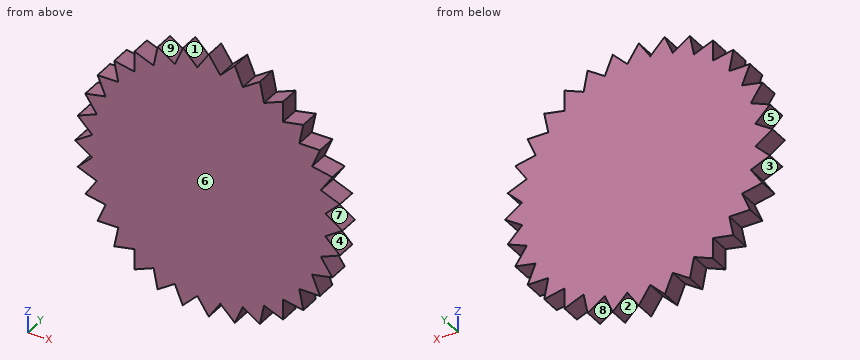
```python
from build123d import *

# Parameters (mm, degrees)
F1_DEPTH = 3.175


with BuildPart() as f1:
    # F0 (on Front) → F1 (new body, symmetric)
    with BuildSketch(Plane.XZ):
        Polygon((-23.3813293569, 34.9926322543), (-23.3813293569, 28.4902322543), (-17.3738950847, 32.5042715037), align=None)
        Polygon((-17.3738950847, 32.5042715037), (-23.3813293569, 28.4902322543), (-28.4902322543, 23.3813293569), (-32.5042715037, 17.3738950847), (-35.2691898278, 10.6987917678), (-36.678732966, 3.6125398832), (-36.678732966, -3.6125398832), (-35.2691898278, -10.6987917678), (-32.5042715037, -17.3738950847), (-28.4902322543, -23.3813293569), (-23.3813293569, -28.4902322543), (-17.3738950847, -32.5042715037), (-10.6987917678, -35.2691898278), (-3.6125398832, -36.678732966), (3.6125398832, -36.678732966), (10.6987917678, -35.2691898278), (17.3738950847, -32.5042715037), (23.3813293569, -28.4902322543), (28.4902322543, -23.3813293569), (32.5042715037, -17.3738950847), (35.2691898278, -10.6987917678), (36.678732966, -3.6125398832), (36.678732966, 3.6125398832), (35.2691898278, 10.6987917678), (32.5042715037, 17.3738950847), (28.4902322543, 23.3813293569), (23.3813293569, 28.4902322543), (17.3738950847, 32.5042715037), (10.6987917678, 35.2691898278), (3.6125398832, 36.678732966), (-3.6125398832, 36.678732966), (-10.6987917678, 35.2691898278), align=None)
        Polygon((-28.4902322543, 23.3813293569), (-23.3813293569, 28.4902322543), (-29.7587875642, 29.7587875642), align=None)
        Polygon((-16.1053397748, 38.881729711), (-17.3738950847, 32.5042715037), (-10.6987917678, 35.2691898278), align=None)
        Polygon((-32.5042715037, 17.3738950847), (-28.4902322543, 23.3813293569), (-34.9926322543, 23.3813293569), align=None)
        Polygon((-8.1233671151, 41.3620697513), (-10.6987917678, 35.2691898278), (-3.6125398832, 36.678732966), align=None)
        Polygon((-35.2691898278, 10.6987917678), (-32.5042715037, 17.3738950847), (-38.881729711, 16.1053397748), align=None)
        Polygon((0, 42.0852809731), (-3.6125398832, 36.678732966), (3.6125398832, 36.678732966), align=None)
        Polygon((-36.678732966, 3.6125398832), (-35.2691898278, 10.6987917678), (-41.2766241, 8.2104310172), align=None)
        Polygon((8.2104310172, 41.2766241), (3.6125398832, 36.678732966), (10.6987917678, 35.2691898278), align=None)
        Polygon((-36.678732966, -3.6125398832), (-36.678732966, 3.6125398832), (-42.0852809731, 0), align=None)
        Polygon((16.1053397748, 38.881729711), (10.6987917678, 35.2691898278), (17.3738950847, 32.5042715037), align=None)
        Polygon((-35.2691898278, -10.6987917678), (-36.678732966, -3.6125398832), (-41.2766241, -8.2104310172), align=None)
        Polygon((23.3813293569, 34.9926322543), (17.3738950847, 32.5042715037), (23.3813293569, 28.4902322543), align=None)
        Polygon((-32.5042715037, -17.3738950847), (-35.2691898278, -10.6987917678), (-38.881729711, -16.1053397748), align=None)
        Polygon((29.7587875642, 29.7587875642), (23.3813293569, 28.4902322543), (28.4902322543, 23.3813293569), align=None)
        Polygon((-28.4902322543, -23.3813293569), (-32.5042715037, -17.3738950847), (-34.9926322543, -23.3813293569), align=None)
        Polygon((34.9926322543, 23.3813293569), (28.4902322543, 23.3813293569), (32.5042715037, 17.3738950847), align=None)
        Polygon((-23.3813293569, -28.4902322543), (-28.4902322543, -23.3813293569), (-29.7587875642, -29.7587875642), align=None)
        Polygon((38.881729711, 16.1053397748), (32.5042715037, 17.3738950847), (35.2691898278, 10.6987917678), align=None)
        Polygon((-17.3738950847, -32.5042715037), (-23.3813293569, -28.4902322543), (-23.3813293569, -34.9926322543), align=None)
        Polygon((41.2766241, 8.2104310172), (35.2691898278, 10.6987917678), (36.678732966, 3.6125398832), align=None)
        Polygon((-10.6987917678, -35.2691898278), (-17.3738950847, -32.5042715037), (-16.1053397748, -38.881729711), align=None)
        Polygon((42.0852809731, 0), (36.678732966, 3.6125398832), (36.678732966, -3.6125398832), align=None)
        Polygon((-3.6125398832, -36.678732966), (-10.6987917678, -35.2691898278), (-8.2104310172, -41.2766241), align=None)
        Polygon((41.2766241, -8.2104310172), (36.678732966, -3.6125398832), (35.2691898278, -10.6987917678), align=None)
        Polygon((3.6125398832, -36.678732966), (-3.6125398832, -36.678732966), (0, -42.0852809731), align=None)
        Polygon((38.881729711, -16.1053397748), (35.2691898278, -10.6987917678), (32.5042715037, -17.3738950847), align=None)
        Polygon((10.6987917678, -35.2691898278), (3.6125398832, -36.678732966), (8.2104310172, -41.2766241), align=None)
        Polygon((34.9926322543, -23.3813293569), (32.5042715037, -17.3738950847), (28.4902322543, -23.3813293569), align=None)
        Polygon((17.3738950847, -32.5042715037), (10.6987917678, -35.2691898278), (16.1053397748, -38.881729711), align=None)
        Polygon((29.7587875642, -29.7587875642), (28.4902322543, -23.3813293569), (23.3813293569, -28.4902322543), align=None)
        Polygon((23.3813293569, -28.4902322543), (17.3738950847, -32.5042715037), (23.3813293569, -34.9926322543), align=None)
    extrude(amount=F1_DEPTH, both=True)


solid = f1.part
```
Here's how the part is built. I have some questions about the finished solid (model axes, mm). Face numbers are marked on the shaded views. A direction names the side the tool comes from. Round coordinates to 2 decimals unless told otherwise and drop trailing zeros. Order: outer loops, then holes, each group sorted by start corner. A loop starts at its lowest first (then second) coordinate and runs counter-clockwise, first axis right, second up. Notation, with made-up numbers: M -24.75,2 L -19.75,2 A9 cw -19.75,11 Z; hole C 71,67.5 d9. An arc over 180 degrees is marked long. One line per question, with ' | ' between items.
1) I want a section at B-B, the plane z = 6. Write out the boundary of the cut face in (x, y) (3 decimals).
Working result:
outline: M -39.066,-3.175 L 39.066,-3.175 L 39.066,3.175 L -39.066,3.175 Z
2) I want a section at A-A, the plane x = -2. Write out the boundary of the cut face in (y, z) (3 decimals).
Working result:
outline: M -3.175,-39.092 L 3.175,-39.092 L 3.175,39.092 L -3.175,39.092 Z
3) I need wall thicknesses on line 1 along Z through (x, y) = (34, -2.5); line 2 along X through (y, z) = (2, 36); line 3 along Z through (x, y) = (-31, -2.75). Which ranges of each line are inside material? Lowest first, please.
Working result:
line 1: -23.38 to -20.98, -17.08 to 17.08, 20.98 to 23.38 | line 2: -16.68 to -11.79, -10.39 to 10.4, 11.79 to 16.68 | line 3: -23.38 to 23.38
4) If we mould it in two halves opening along Z, with no side actions, what happens to the marked faces 1, 2, 3 and 4? For each: +Z half, -Z half, draft (parallel to the pull), parting line (faces both ways), or undercut.
Working result:
face 1: +Z half | face 2: -Z half | face 3: undercut | face 4: undercut
5) For pin 1 Ø3 at (y, z) = (-1.5, 31) entering from +X; pin 2 Ø1.9 at (x, y) = (31.5, 1) entering from -Z; pin 3 Ø1 at (x, y) = (13, -1.5) entering from +Z, each with a flat end and sliding along its axis, tell me the tip position at first contact or that it passes through.
Working result:
pin 1: x = 29.76 | pin 2: z = -23.38 | pin 3: z = 37.14
6) For the marked faces 5, 6, 7, 8 and 9, which set-ups out of +Z, -Z, +X, -X, +Y, -Y let a thin tool reach every point of the face, with its end or its side?
Working result:
face 5: -X, +Y, -Y | face 6: +Z, -Z, +X, -X, -Y | face 7: +X, +Y, -Y | face 8: -Z, +Y, -Y | face 9: +Z, +Y, -Y
